from build123d import *

# Parameters (mm, degrees)
F1_DEPTH = 38.1


with BuildPart() as f1:
    # F0 (on Front) → F1 (new body)
    with BuildSketch(Plane.XZ):
        with BuildLine():
            Line((23.746809, 23.746809), (3.054569, 25.323361))
            ThreePointArc((3.054569, 25.323361), (-20.828977, 21.67196), (-42.665429, 11.331465))
            ThreePointArc((-42.665429, 11.331465), (-57.594957, 11.552189), (-72.225779, 8.5725))
            Line((-72.225779, 8.5725), (-79.409733, 4.488737))
            Line((-79.409733, 4.488737), (-82.107544, 2.463362))
            Line((-82.107544, 2.463362), (-77.172592, 0))
            Line((-77.172592, 0), (-73.197633, -1.392897))
            Line((-73.197633, -1.392897), (-78.291319, -4.039914))
            Line((-78.291319, -4.039914), (-67.496121, -4.039914))
            Line((-67.496121, -4.039914), (-61.978191, -4.039914))
            ThreePointArc((-61.978191, -4.039914), (-53.701295, 5.423382), (-45.424398, -4.039914))
            Line((-45.424398, -4.039914), (49.562849, -4.039914))
            ThreePointArc((49.562849, -4.039914), (55.005727, 7.621836), (66.707842, 2.266293))
            Line((66.707842, 2.266293), (66.707842, 6.207672))
            Line((66.707842, 6.207672), (66.707842, 17.440604))
            Line((66.707842, 17.440604), (62.779258, 14.65251))
            Line((62.779258, 14.65251), (59.81043, 14.878707))
            Line((59.81043, 14.878707), (41.483015, 20.199569))
            Line((41.483015, 20.199569), (23.746809, 23.746809))
        make_face()
    extrude(amount=F1_DEPTH)


solid = f1.part
CAD build for the part. Positions are in the model's coordinates, mm. A direction names the side the tool comes from. Coordinates: 2 decimals unless noted, no trailing zeros. Order: outer loops, then holes, each group sorted by start corner. A loop starts at its lowest first (then second) coordinate and runs counter-clockwise, first axis right, second up. Notation, with made-up numbers: (5.5, 8) -> (23.5, 8) arc R19 cw to (23.5, 22) -> close; hole circle Ø6 at (0, 10.25). An arc over 180 degrees is marked (long way). Answer in a Markdown table with one row per item.
1) Mould opens along X. For faces 4 (the face through (61.316, -18.783, 14.764)), 5 (the face through (54.82, -18.78, 7.55)), 6 (the face through (-9, -38.1, 8)), 7 (the face through (66.708, -19, 10)) say: pulls with the +X half, pulls with the -X half, needs draft (parallel to the pull), parting line crosses it, or undercut.
Check values:
| item | result |
|---|---|
| face 4 | undercut |
| face 5 | undercut |
| face 6 | needs draft |
| face 7 | pulls with the +X half |
2) Band-saw the part on B-B (z = 22). List the corners of the cut face in (x, y).
Check values:
| item | result |
|---|---|
| outline | (-19.73, -38.1) -> (32.48, -38.1) -> (32.48, 0) -> (-19.73, 0) -> close |
3) Band-saw the part on A-A (y = -36). List the corners of the cut face in (x, z), and give its area (3 significant figures).
Check values:
| item | result |
|---|---|
| outline | (-82.11, 2.46) -> (-77.17, 0) -> (-73.2, -1.39) -> (-78.29, -4.04) -> (-61.98, -4.04) arc R8.35 cw (long way) to (-45.42, -4.04) -> (49.56, -4.04) arc R9.13 cw to (66.71, 2.27) -> (66.71, 17.44) -> (62.78, 14.65) -> (59.81, 14.88) -> (41.48, 20.2) -> (23.75, 23.75) -> (3.05, 25.32) arc R83.45 ccw to (-42.67, 11.33) arc R69.36 ccw to (-72.23, 8.57) -> (-79.41, 4.49) -> close |
| area | 2,910 mm2 |
4) Which spindle directions (+Z, -Z, +X, -X, +Y, -Y) get a long thin tool onto all of the face, cutting with end or side? Do faces 1 (the face through (-79.675, -18.783, 1.249)), 2 (the face through (13.546, -18.783, 24.524)), 3 (the face through (64.771, -18.783, 16.066)). Say none if no direction does.
Check values:
| item | result |
|---|---|
| face 1 | -X, +Y, -Y |
| face 2 | +Z, +X, +Y, -Y |
| face 3 | +Z, +Y, -Y |
5) Drill centre lines: line 1 (X direction, y = -9.5, z = 4.25); line 2 (X direction, y = -18.5, z = -2); line 3 (X direction, y = -12, z = 6.25). Where is each one in solid material? Low to high.
Check values:
| item | result |
|---|---|
| line 1 | -79.73 to -57.97, -49.43 to 50.65, 65.67 to 66.71 |
| line 2 | -74.37 to -62, -45.4 to 49.09 |
| line 3 | -76.31 to 52.54, 63.78 to 66.71 |
6) Band-saw the part on C-C (x = -11). List the corners of the cut face in (y, z), and give its area (3 significant figures).
Check values:
| item | result |
|---|---|
| outline | (-38.1, -4.04) -> (0, -4.04) -> (0, 24.04) -> (-38.1, 24.04) -> close |
| area | 1,070 mm2 |
7) Flat gauge pins, fed straight in: P1, Ø2, axis at y = -14, z = 6.5, coming from the -X side; P2, Ø10, axis at x = 24.5, z = 5, coming from the +Y side; P3, Ø10, axis at x = -53.7, z = -2.93, coming from the -Y side; P4, Ø2, axis at x = -27, y = -28.5, coming from the +Z side. Where does each tip first touch, or does it go through?
Check values:
| item | result |
|---|---|
| P1 | x = -77.63 |
| P2 | y = 0 |
| P3 | through |
| P4 | z = 19.9 |
